Here's how the part is built. I have some questions about the finished solid (model axes, mm). A direction names the side the tool comes from. Round coordinates to 2 decimals unless told otherwise and drop trailing zeros. Write each loop counter-clockwise with the first axis right and the second up, starting at its lowest first coordinate (ties: lowest second). Pieces come first, ordered by that corner, then holes. Notation, with made-up numbers: (62.5, -1.5) -> (90.5, -1.5) arc R14 ccw to (90.5, 23.5) -> close; hole circle Ø5 at (49, 54). An arc over 180 degrees is marked (long way). Answer in a Markdown table with one row per item. Add a question column.
from build123d import *

# Parameters (mm, degrees)
SKETCH1_W           = 7
SKETCH1_H           = 7
BOSS_EXTRUDE1_DEPTH = 3
CUT_EXTRUDE1_DEPTH  = 7
CUT_EXTRUDE2_DEPTH  = 11
SKETCH4_R           = 1.8
CUT_EXTRUDE3_DEPTH  = 0.8
CUT_EXTRUDE4_DEPTH  = 0.4


with BuildPart() as part:
    # Sketch1 → Boss-Extrude1 (new body)
    with BuildSketch(Plane(origin=(0, 0, 0), x_dir=(1, 0, 0), z_dir=(0, 1, 0))):
        with Locations((3.5, 3.5)):
            Rectangle(SKETCH1_W, SKETCH1_H)
    extrude(amount=BOSS_EXTRUDE1_DEPTH)

    # Sketch2 → Cut-Extrude1 (cut)
    with BuildSketch(Plane.XY):
        Polygon((0, 0), (0.7, 3), (0, 3), align=None)
        Polygon((7, 0), (6.3, 3), (7, 3), align=None)
    extrude(amount=-CUT_EXTRUDE1_DEPTH, mode=Mode.SUBTRACT)

    # Sketch3 → Cut-Extrude2 (cut)
    with BuildSketch(Plane(origin=(0, 0, 0), x_dir=(0, 0, -1), z_dir=(1, 0, 0))):
        Polygon((0, 0), (0.7, 3), (0, 3), align=None)
        Polygon((7, 3), (6.3, 3), (7, 0), align=None)
    extrude(amount=CUT_EXTRUDE2_DEPTH, mode=Mode.SUBTRACT)

    # Sketch4 → Cut-Extrude3 (cut)
    with BuildSketch(Plane.XZ):
        with Locations(Location((3.5, -3.5, 0), (0, 0, 270))):
            Circle(SKETCH4_R)
    extrude(amount=-CUT_EXTRUDE3_DEPTH, mode=Mode.SUBTRACT)

    # Sketch5 → Cut-Extrude4 (cut)
    with BuildSketch(Plane(origin=(0, 3, 0), x_dir=(1, 0, 0), z_dir=(0, 1, 0))):
        Polygon((5.198883611, 1.79301719), (4.485141624, 1.79301719), (4.189969348, 2.600709497), (2.846619989, 2.600709497), (2.551447713, 1.79301719), (1.833498995, 1.79301719), (3.156515822, 5.29301719), (3.869556688, 5.29301719), align=None)
        Polygon((3.976127201, 3.184042831), (3.516191303, 4.440453087), (3.057657649, 3.184042831), align=None, mode=Mode.SUBTRACT)
    extrude(amount=-CUT_EXTRUDE4_DEPTH, mode=Mode.SUBTRACT)


solid = part.part
Item 1: For P1, Ø1.5, axis at y = 1.5, z = -3.5, coming from the +X side (3 decimals), with a flat end and sliding along its axis, tell me the tip position at first contact or that it passes through.
Item 2: On a 3-axis mill with a long thin cutter (end or side, diameter ignored), from which of +Z, -Z, +X, -X, +Y, -Y can I reach the whole of each face in a straight line? I mean faces 5 (the flat face through (3.451, 1.521, -6.645)), 6 (the flat face through (4, 0.8, -3)), 7 (the flat face through (2.486, 2.803, -3.519)). Say none if no direction works.
Item 3: If we section it at D-D on z = -1.5: Please give me the cut outline in (x, y), then the cut area to 3 significant figures.
Item 4: I need wall thicknesses on line 1 along Y through (x, z) = (4.25, -2); line 2 along X through (y, z) = (0.3, -3.5); line 3 along X through (y, z) = (0.2, -3.5). Which ranges of each line are inside material? Lowest first, please. Write a range as from..to.
Item 5: If we section it at B-B on z = -3.5: Please give me the cut outline in (x, y).
Item 6: If we section it at C-C on x = 1.25: Please give me the cut outline in (y, z).
Item 7: If we section it at A-A on y = 0.3: Please give me the cut outline in (x, z), then the cut area to 3 significant figures.
Item 8: If we mould it in two halves opening along X, with no side actions, what happens to faces 1 (the flat face through (0.345, 1.479, -3.451)), 2 (the flat face through (4, 2.6, -3)), 3 (the cylindrical face through (4.041, 0.394, -5.217)), 4 (the flat face through (2, 0, -5))? For each: pulls with the +X half, pulls with the -X half, needs draft (parallel to the pull), parting line crosses it, or undercut.
Results list:
| question | item | result |
|---|---|---|
| 1 | P1 | x = 6.825 |
| 2 | face 5 | -Z, +X, -X, +Y |
| 2 | face 6 | -Y |
| 2 | face 7 | +Y |
| 3 | outline | (0, 0) -> (7, 0) -> (6.3, 3) -> (0.7, 3) -> close |
| 3 | area | 18.9 mm² |
| 4 | line 1 | 0.8..3 |
| 4 | line 2 | 0.07..1.7, 5.3..6.93 |
| 4 | line 3 | 0.05..1.7, 5.3..6.95 |
| 5 | outline | (0, 0) -> (1.7, 0) -> (1.7, 0.8) -> (5.3, 0.8) -> (5.3, 0) -> (7, 0) -> (6.3, 3) -> (4.55, 3) -> (4.55, 2.6) -> (3.86, 2.6) -> (3.86, 3) -> (3.17, 3) -> (3.17, 2.6) -> (2.48, 2.6) -> (2.48, 3) -> (0.7, 3) -> close |
| 6 | outline | (0, -7) -> (3, -6.3) -> (3, -0.7) -> (0, 0) -> close |
| 7 | outline | (0.07, -6.93) -> (6.93, -6.93) -> (6.93, -0.07) -> (0.07, -0.07) -> close; hole circle Ø3.6 at (3.5, -3.5) |
| 7 | area | 36.9 mm² |
| 8 | face 1 | pulls with the -X half |
| 8 | face 2 | undercut |
| 8 | face 3 | undercut |
| 8 | face 4 | needs draft |
